Can you work these out from the model? Positions are in its coordinate system, mm. Round coordinates to 2 decimals unless told otherwise and drop trailing zeros. Loops run counter-clockwise (first coordinate to the right, second up) from the corner with the lowest first, then second, coordinate; pieces in that order, holes last. Notation, with made-up numbers: M -25.5,52.5 L -17.5,52.5 A4 ccw -17.5,59.5 Z; hole C 23,84.5 d9. An arc over 180 degrees is marked long. Return JSON: item names as keys, results as strings.
Autodesk Inventor part; units mm, degrees
ref_plane "YZ Plane" through (0, 0, 0) normal (1, 0, 0) x (0, 1, 0)
ref_plane "XZ Plane" through (0, 0, 0) normal (0, 1, 0) x (-1, 0, 0)
ref_plane "XY Plane" through (0, 0, 0) normal (0, 0, 1) x (1, 0, 0)
sketch "Sketch1" plane through (0, 0, 0) normal (0, 0, 1) x (1, 0, 0)
  line L0 (-21.273, 9.4908) -> (-21.273, -38.5092)
  line L1 (-21.273, -38.5092) -> (13.727, -38.5092)
  line L2 (66.227, -35.5092) -> (66.227, 6.4908)
  line L3 (-21.273, 9.4908) -> (13.727, 9.4908)
  line L4 (13.727, 9.4908) -> (13.727, 6.4908)
  line L5 (13.727, 6.4908) -> (66.227, 6.4908)
  line L6 (13.727, 6.4908) -> (13.727, -38.5092)
  line L7 (66.227, -35.5092) -> (13.727, -35.5092)
  line L8 (13.727, -38.5092) -> (66.227, -35.5092)
  line L9 (66.227, 6.4908) -> (13.727, 9.4908)
  point P0 (0, 0)
  point P1 (-16.273, 4.9908)
  point P2 (-16.273, -14.5092)
  point P3 (-16.273, -34.0092)
  point P4 (8.727, 4.9908)
  point P5 (8.727, -14.5092)
  point P6 (8.727, -34.0092)
  point P7 (29.727, 0.9908)
  point P8 (29.727, -30.0092)
  point P9 (60.727, -30.0092)
  point P10 (60.727, 0.9908)
  point P11 (45.227, -14.5092)
  dimension "d0" = 48
  dimension "d2" = 42
  dimension "d3" = 35
  dimension "d4" = 5
  dimension "d5" = 5
  dimension "d6" = 4.5
  dimension "d7" = 4.5
  dimension "d8" = 24
  dimension "d9" = 31
  dimension "d10" = 31
  dimension "d13" = 15.5
  dimension "d14" = 15.5
  dimension "d44" = 5.5
  dimension "d45" = 87.5
  dimension "d46" = 5.5
  dimension "d47" = 3
  dimension "d52" = 52.5
extrude "Extrusion1" add sketch "Sketch1" along normal blind 2.5
hole "Hole1" at (-16.273, 4.9908, 0) at (-16.273, -14.5092, 0) at (-16.273, -34.0092, 0) at (8.727, 4.9908, 0) at (8.727, -14.5092, 0) at (8.727, -34.0092, 0) direction (0, 0, 1) diameter 3 end through all
hole "Hole2" at (29.727, 0.9908, 0) at (29.727, -30.0092, 0) at (60.727, -30.0092, 0) at (60.727, 0.9908, 0) direction (0, 0, 1) diameter 2.5 end through all
hole "Hole3" at (45.227, -14.5092, 0) direction (0, 0, 1) diameter 22 end through all
chamfer "Chamfer3" distance 3 angle 45 2 edges at (-21.273, -38.5092, 1.25) (-21.273, 9.4908, 1.25)
equation "\"d47\" = -0.5 * d2 + 0.5 * d0"
properties part number "LC_ALU_3mm_X_axis_stepper_mount_plate" material "Aluminum 6061-AHC"
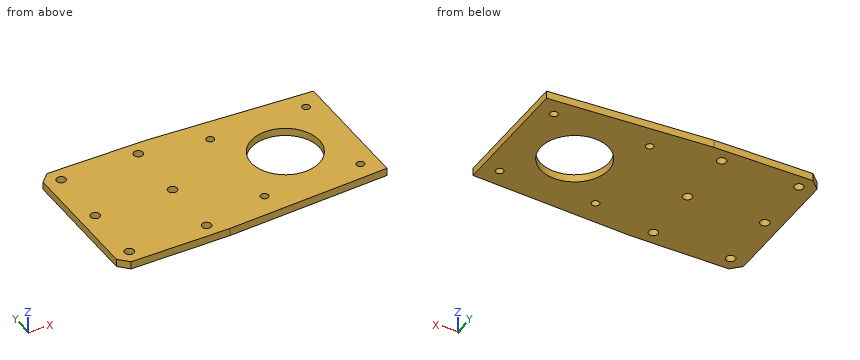
Q1. If I drill on line 1 along X through (y, z) = (-29, 0.3); line 2 along X through (y, z) = (4, 1.15); line 3 along X through (y, z) = (-15, 2), over which ranges is the centre line in solid material (lowest first)?
Results:
{"line 1": "x = -21.27 to 28.99, 30.46 to 59.99, 61.46 to 66.23", "line 2": "x = -21.27 to -17.4, -15.15 to 7.6, 9.85 to 66.23", "line 3": "x = -21.27 to -17.69, -14.86 to 7.31, 10.14 to 34.24, 56.22 to 66.23"}
Q2. Suppose I cut it at A-A, the plane x = 40.5. Please give me the cut outline in (y, z), plus the area to 3 significant figures.
Results:
{"outline": "M -36.98,0 L -24.44,0 L -24.44,2.5 L -36.98,2.5 Z; M -4.58,0 L 7.96,0 L 7.96,2.5 L -4.58,2.5 Z", "area": "62.7 mm2"}
Q3. Suppose I cut it at D-D, the plane x = 22.5. Please give me the cut outline in (y, z), plus the area to 3 significant figures.
Results:
{"outline": "M -38.01,0 L 8.99,0 L 8.99,2.5 L -38.01,2.5 Z", "area": "117 mm2"}
Q4. Suppose I cut it at C-C, the plane y = -24. Please give me the cut outline in (x, z), plus the area to 3 significant figures.
Results:
{"outline": "M -21.27,0 L 39.67,0 L 39.67,2.5 L -21.27,2.5 Z; M 50.79,0 L 66.23,0 L 66.23,2.5 L 50.79,2.5 Z", "area": "191 mm2"}
Q5. Suppose I cut it at B-B, the plane z = 1.2. State how many separate pieces and enclosed holes the cut face has, plus the area to 3 significant figures.
Results:
{"separate pieces": "1", "enclosed holes": "11", "area": "3,590 mm2"}
